```python
from build123d import *

# Parameters (mm, degrees)
SKIZZE1_R                       = 6
AUFSATZ_LINEAR_AUSTRAGEN1_DEPTH = 9
SKIZZE2_R                       = 3.925
AUFSATZ_LINEAR_AUSTRAGEN2_DEPTH = 41
SKIZZE3_R                       = 21
AUFSATZ_LINEAR_AUSTRAGEN3_DEPTH = 19
SKIZZE4_R                       = 6.075
SCHNITT_LINEAR_AUSTRAGEN2_DEPTH = 10
VERRUNDUNG1_R                   = 2
SKIZZE5_R                       = 1.5
SCHNITT_LINEAR_AUSTRAGEN3_DEPTH = 15


with BuildPart() as part:
    # Skizze1 → Aufsatz-Linear austragen1 (new body)
    with BuildSketch(Plane.XY):
        Circle(SKIZZE1_R)
    extrude(amount=AUFSATZ_LINEAR_AUSTRAGEN1_DEPTH)

    # Skizze2 → Aufsatz-Linear austragen2 (add)
    with BuildSketch(Plane(origin=(0, 0, 0), x_dir=(-1, 0, 0), z_dir=(0, 0, -1))):
        Circle(SKIZZE2_R)
    extrude(amount=AUFSATZ_LINEAR_AUSTRAGEN2_DEPTH)

    # Skizze3 → Aufsatz-Linear austragen3 (add)
    with BuildSketch(Plane.XY.offset(9)):
        Circle(SKIZZE3_R)
    extrude(amount=AUFSATZ_LINEAR_AUSTRAGEN3_DEPTH)

    # Skizze4 → Schnitt-Linear austragen2 (cut)
    with BuildSketch(Plane.XY.offset(28)):
        Circle(SKIZZE4_R)
    extrude(amount=-SCHNITT_LINEAR_AUSTRAGEN2_DEPTH, mode=Mode.SUBTRACT)

    # Verrundung1
    verrundung1_edges = [part.edges().sort_by_distance(p)[0] for p in [
        (-6.075, 0, 28),
    ]]
    fillet(verrundung1_edges, radius=VERRUNDUNG1_R)

    # Skizze5 → Schnitt-Linear austragen3 (cut)
    with BuildSketch(Plane(origin=(0, 0, -41), x_dir=(-1, 0, 0), z_dir=(0, 0, -1))):
        Circle(SKIZZE5_R)
    extrude(amount=-SCHNITT_LINEAR_AUSTRAGEN3_DEPTH, mode=Mode.SUBTRACT)


solid = part.part
```
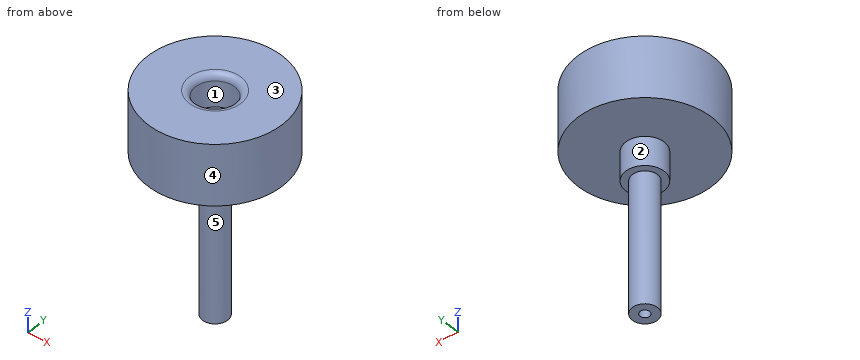
Here's how the part is built. I have some questions about the finished solid (model axes, mm). Face numbers are marked on the shaded views. A direction names the side the tool comes from. Coordinates: 2 decimals unless noted, no trailing zeros. Order: outer loops, then holes, each group sorted by start corner. A loop starts at its lowest first (then second) coordinate and runs counter-clockwise, first axis right, second up. Notation, with made-up numbers: (13, 58) - (36, 58) arc R17 ccw to (36, 82) - close; hole circle Ø9 at (56.25, -20). An arc over 180 degrees is marked (long way). One line per question, with ' | ' between items.
(1) Suppose I cut it at A-A on x = 0. List the corners of the cut face in (y, z) for me (3 decimals).
Report:
outline: (-21, 9) - (-6, 9) - (-6, 0) - (-3.925, 0) - (-3.925, -41) - (-1.5, -41) - (-1.5, -26) - (1.5, -26) - (1.5, -41) - (3.925, -41) - (3.925, 0) - (6, 0) - (6, 9) - (21, 9) - (21, 28) - (8.075, 28) arc R2 ccw to (6.075, 26) - (6.075, 18) - (-6.075, 18) - (-6.075, 26) arc R2 ccw to (-8.075, 28) - (-21, 28) - close
(2) If we mould it in two halves opening along X, with no side actions, what happens to the marked faces 1, 2 and 3? For each: pulls with the +X half, pulls with the -X half, needs draft (parallel to the pull), parting line crosses it, or undercut.
Report:
face 1: undercut | face 2: parting line crosses it | face 3: needs draft
(3) For the marked faces 4 and 5, which set-ups out of +Z, -Z, +X, -X, +Y, -Y let a thin tool reach every point of the face, with its end or its side?
Report:
face 4: +Z, -Z | face 5: -Z
(4) Suppose I cut it at C-C on z = 17. List the corners of the cut face in (x, y) for me.
Report:
outline: circle Ø42 at (0, 0)
(5) If I drill on L1, parallel to Y at x = 0, z = 21 (3 decimals); L2, parallel to Y at x = 0, z = -31 (3 decimals); L3, parallel to Z at x = 5, y = 16, over which ranges is the centre line in solid material (lowest first)?
Report:
L1: y = -21 to -6.075, 6.075 to 21 | L2: y = -3.925 to -1.5, 1.5 to 3.925 | L3: z = 9 to 28
(6) Will these pins go through, and if not, where does the flat tip stop? pin 1 (1.8 mm diameter, centred on x = 0, y = 0, fed in from -Z); pin 2 (3 mm diameter, centred on x = -16.5, y = -8, fed in from -Z); pin 3 (3 mm diameter, centred on y = 5, z = 4.5, fed in from -X).
Report:
pin 1: stops at z = -26 | pin 2: stops at z = 9 | pin 3: stops at x = -4.87
(7) Suppose I cut it at D-D on y = 9. List the corners of the cut face in (x, z) for me, and give its area (3 significant figures).
Report:
outline: (-18.97, 9) - (18.97, 9) - (18.97, 28) - (-18.97, 28) - close | area: 721 mm2
